Here's how the part is built. I have some questions about the finished solid (model axes, mm). A direction names the side the tool comes from. Coordinates: 2 decimals unless noted, no trailing zeros. Order: outer loops, then holes, each group sorted by start corner. A loop starts at its lowest first (then second) coordinate and runs counter-clockwise, first axis right, second up.
```python
from build123d import *

# Parameters (mm, degrees)
SKETCH1_R           = 1.6
BOSS_EXTRUDE1_DEPTH = 5
BOSS_EXTRUDE5_DEPTH = 20
FILLET8_R           = 34
FILLET9_R           = 37
REVOLVE4_ANGLE      = 90
BOSS_EXTRUDE6_DEPTH = 20
CUT_EXTRUDE3_REACH  = 593.738
SKETCH16_W          = 40
SKETCH16_H          = 5
FILLET10_R          = 22
CUT_EXTRUDE4_REACH  = 581.899
SKETCH17_R          = 7.5
FILLET11_R          = 5
FILLET12_R          = 2
CUT_EXTRUDE5_REACH  = 581.899
SKETCH18_R          = 3
SKETCH19_W          = 201.306473633
SKETCH19_H          = 285.537776223
CUT_EXTRUDE6_DEPTH  = 269
FILLET13_R          = 7


with BuildPart() as part:
    # Sketch1 → Boss-Extrude1 (new body)
    with BuildSketch(Plane(origin=(0, 0, 0), x_dir=(1, 0, 0), z_dir=(0, 1, 0))):
        Polygon((-165, 270), (-165, -270), (0, -270), (0, -254), (-149, -254), (-149, 254), (0, 254), (0, 270), align=None)
        with Locations(Location((-159, 130, 0), (0, 0, 270))):
            Circle(SKETCH1_R, mode=Mode.SUBTRACT)
        with Locations(Location((-159, 50, 0), (0, 0, 270))):
            Circle(SKETCH1_R, mode=Mode.SUBTRACT)
        with Locations(Location((-120, 264, 0), (0, 0, 270))):
            Circle(SKETCH1_R, mode=Mode.SUBTRACT)
        with Locations(Location((-40, 264, 0), (0, 0, 270))):
            Circle(SKETCH1_R, mode=Mode.SUBTRACT)
        with Locations(Location((-159, 210, 0), (0, 0, 270))):
            Circle(SKETCH1_R, mode=Mode.SUBTRACT)
        with Locations(Location((-40, -264, 0), (0, 0, 90))):
            Circle(SKETCH1_R, mode=Mode.SUBTRACT)
        with Locations(Location((-120, -264, 0), (0, 0, 90))):
            Circle(SKETCH1_R, mode=Mode.SUBTRACT)
        with Locations(Location((-159, -210, 0), (0, 0, 90))):
            Circle(SKETCH1_R, mode=Mode.SUBTRACT)
        with Locations(Location((-159, -50, 0), (0, 0, 90))):
            Circle(SKETCH1_R, mode=Mode.SUBTRACT)
        with Locations(Location((-159, -130, 0), (0, 0, 90))):
            Circle(SKETCH1_R, mode=Mode.SUBTRACT)
    extrude(amount=BOSS_EXTRUDE1_DEPTH)

    # Sketch12 → Boss-Extrude5 (add)
    with BuildSketch(Plane(origin=(0, 5, 0), x_dir=(1, 0, 0), z_dir=(0, 1, 0))):
        Polygon((0, 254), (-149, 254), (-149, -254), (0, -254), (0, -257), (-152, -257), (-152, 257), (0, 257), align=None)
    extrude(amount=BOSS_EXTRUDE5_DEPTH)

    # Fillet8
    fillet8_edges = [part.edges().sort_by_distance(p)[0] for p in [
        (-149, 12.5, -254),
        (-149, 12.5, 254),
    ]]
    fillet(fillet8_edges, radius=FILLET8_R)

    # Fillet9
    fillet9_edges = [part.edges().sort_by_distance(p)[0] for p in [
        (-152, 15, -257),
        (-152, 15, 257),
    ]]
    fillet(fillet9_edges, radius=FILLET9_R)

    # Sketch13 → Revolve4 (revolve)
    with BuildSketch(Plane(origin=(0, 25, 0), x_dir=(1, 0, 0), z_dir=(0, 1, 0))):
        with BuildLine():
            Line((0, 254), (-115, 254))
            ThreePointArc((-115, 254), (-139.04163056, 244.04163056), (-149, 220))
            Line((-149, 220), (-149, -220))
            ThreePointArc((-149, -220), (-139.04163056, -244.04163056), (-115, -254))
            Line((-115, -254), (0, -254))
            Line((0, -254), (0, -257))
            Line((0, -257), (-115, -257))
            ThreePointArc((-115, -257), (-141.162950904, -246.162950904), (-152, -220))
            Line((-152, -220), (-152, 220))
            ThreePointArc((-152, 220), (-141.162950904, 246.162950904), (-115, 257))
            Line((-115, 257), (0, 257))
            Line((0, 257), (0, 254))
        make_face()
    revolve(axis=Axis((0, 25, -257), (0, 0, -1)), revolution_arc=REVOLVE4_ANGLE)

    # Sketch15 → Boss-Extrude6 (add)
    with BuildSketch(Plane(origin=(0, 0, 0), x_dir=(0, 0, -1), z_dir=(1, 0, 0))):
        with BuildLine():
            Line((-254, 5), (-254, 140))
            ThreePointArc((-254, 140), (-244.04163056, 164.04163056), (-220, 174))
            Line((-220, 174), (220, 174))
            ThreePointArc((220, 174), (244.04163056, 164.04163056), (254, 140))
            Line((254, 140), (254, 5))
            Line((254, 5), (254, 0))
            Line((254, 0), (270, 0))
            Line((270, 0), (270, 5))
            Line((270, 5), (257, 5))
            Line((257, 5), (257, 140))
            ThreePointArc((257, 140), (246.162950904, 166.162950904), (220, 177))
            Line((220, 177), (-220, 177))
            ThreePointArc((-220, 177), (-246.162950904, 166.162950904), (-257, 140))
            Line((-257, 140), (-257, 5))
            Line((-257, 5), (-270, 5))
            Line((-270, 5), (-270, 0))
            Line((-270, 0), (-254, 0))
            Line((-254, 0), (-254, 5))
        make_face()
    extrude(amount=BOSS_EXTRUDE6_DEPTH)

    # Cut-Extrude3: up to this face of the body (flat: up to its plane)
    cut_extrude3_end = Plane(part.part.faces().sort_by_distance((-72.5, 2.5, -270))[0])
    # Sketch16 → Cut-Extrude3 (cut, up to the picked face)
    with BuildSketch(Plane.XY.offset(270), mode=Mode.PRIVATE) as cut_extrude3_sk1:
        with Locations((0, 2.5)):
            Rectangle(SKETCH16_W, SKETCH16_H)
    cut_extrude3_tool1 = split(extrude(cut_extrude3_sk1.sketch, amount=-CUT_EXTRUDE3_REACH, mode=Mode.PRIVATE), bisect_by=cut_extrude3_end, keep=Keep.BOTH, mode=Mode.PRIVATE)
    add(cut_extrude3_tool1.solids().sort_by(Axis((0, 2.5, 270), (0, 0, -1)))[0], mode=Mode.SUBTRACT)

    # Fillet10
    fillet10_edges = [part.edges().sort_by_distance(p)[0] for p in [
        (20, 5, 255.5),
        (20, 5, -255.5),
    ]]
    fillet(fillet10_edges, radius=FILLET10_R)

    # Cut-Extrude4: up to this face of the body (flat: up to its plane)
    cut_extrude4_end = Plane(part.part.faces().sort_by_distance((-40.16059182, 65.16059182, -257))[0])
    # Sketch17 → Cut-Extrude4 (cut, up to the picked face)
    with BuildSketch(Plane.XY.offset(257), mode=Mode.PRIVATE) as cut_extrude4_sk1:
        with Locations((0, 25)):
            Circle(SKETCH17_R)
    cut_extrude4_tool1 = split(extrude(cut_extrude4_sk1.sketch, amount=-CUT_EXTRUDE4_REACH, mode=Mode.PRIVATE), bisect_by=cut_extrude4_end, keep=Keep.BOTH, mode=Mode.PRIVATE)
    add(cut_extrude4_tool1.solids().sort_by(Axis((0, 25, 257), (0, 0, -1)))[0], mode=Mode.SUBTRACT)

    # Fillet11
    fillet11_edges = [part.edges().sort_by_distance(p)[0] for p in [
        (-165, 2.5, 270),
        (-165, 2.5, -270),
    ]]
    fillet(fillet11_edges, radius=FILLET11_R)

    # Fillet12
    fillet12_edges = [part.edges().sort_by_distance(p)[0] for p in [
        (-152, 5, 0),
        (-67.5, 5, 257),
        (-141.162950904, 5, -246.162950904),
        (-141.162950904, 5, 246.162950904),
        (-67.5, 5, -257),
    ]]
    fillet(fillet12_edges, radius=FILLET12_R)

    # Cut-Extrude5: up to this face of the body (flat: up to its plane)
    cut_extrude5_end = Plane(part.part.faces().sort_by_distance((-40.288135092, 66.389949232, 257))[0])
    # Sketch18 → Cut-Extrude5 (cut, up to the picked face)
    with BuildSketch(Plane(origin=(0, 0, -257), x_dir=(-1, 0, 0), z_dir=(0, 0, -1)), mode=Mode.PRIVATE) as cut_extrude5_sk1:
        with Locations((99.306112319, 13.240065646)):
            Circle(SKETCH18_R)
    cut_extrude5_tool1 = split(extrude(cut_extrude5_sk1.sketch, amount=-CUT_EXTRUDE5_REACH, mode=Mode.PRIVATE), bisect_by=cut_extrude5_end, keep=Keep.BOTH, mode=Mode.PRIVATE)
    add(cut_extrude5_tool1.solids().sort_by(Axis((-99.306112, 13.240066, -257), (0, 0, 1)))[0], mode=Mode.SUBTRACT)

    # Sketch19 → Cut-Extrude6 (cut)
    with BuildSketch(Plane.XZ):
        with Locations((-80.653236817, -142.768888112)):
            Rectangle(SKETCH19_W, SKETCH19_H)
    extrude(amount=-CUT_EXTRUDE6_DEPTH, mode=Mode.SUBTRACT)

    # Fillet13
    fillet13_edges = [part.edges().sort_by_distance(p)[0] for p in [
        (20, 175.5, 0),
    ]]
    fillet(fillet13_edges, radius=FILLET13_R)


solid = part.part
```
Q1. Will these pins go through, and if not, where does the flat tip stop? pin 1 (6 mm diameter, centred on x = -5, z = 90.5, fed in from -Y); pin 2 (8 mm diameter, centred on x = -99.31, y = 13.24, fed in from -Z); pin 3 (6 mm diameter, centred on x = 10.5, z = 154, fed in from -Y).
Q2. We'd pull the mould along X, two halves only. Please class faces 1 (the flat face through (-152, 0, 186)), 2 (the cylindrical face through (-97.095, 15.268, 255.479)), 3 (the cylindrical face through (-106.511, 129.194, 111.54)), 4 (the cylindrical face through (-0.976, 32.436, 255.521)): pulls with the +X half, pulls with the -X half, needs draft (parallel to the pull), parting line crosses it, or undercut.
Q3. I need wall thicknesses on L1, parallel to Z at x = -159, y = 3.45; L2, parallel to X at y = 1.5, z = 50; L3, parallel to X at y = 3.7, z = 264. Which ranges of each line are inside material? Lowest first, please.
Q4. If we section it at A-A on z = 168: Write out the boundary of the cut face in (x, y).
Q5. For faces 5 (the flat face through (20, 175, 123)), 6 (the flat face through (-157, 5, 184)), 7 (the flat face through (-152, 16, 112)), 8 (the flat face through (-149, 12, 108)), which set-ups out of +Z, -Z, +X, -X, +Y, -Y let a thin tool reach every point of the face, with its end or its side?
Reply:
1. pin 1: stops at y = 173.79
1. pin 2: stops at z = 254
1. pin 3: stops at y = 174
2. face 1: needs draft
2. face 2: undercut
2. face 3: pulls with the +X half
2. face 4: undercut
3. L1: z = 0 to 48.4, 51.6 to 128.4, 131.6 to 208.4, 211.6 to 270
3. L2: x = -165 to -160.6, -157.4 to -149
3. L3: x = -165 to -121.6, -118.4 to -41.6, -38.4 to -20
4. outline: (-165, 0) - (-149, 0) - (-149, 25) arc R149 cw to (0, 174) - (20, 174) - (20, 177) - (0, 177) arc R152 ccw to (-152, 25) - (-152, 7) arc R2 cw to (-154, 5) - (-165, 5) - close
5. face 5: +Z, -Z, +X, +Y, -Y
5. face 6: +Z, -X, +Y
5. face 7: +Z, -Z, -X, +Y
5. face 8: -Z, +X, -Y
